```python
from build123d import *

# Parameters (mm, degrees)
EXTRUDE_1_DEPTH          = 99
CUT_EXTRUDE_1_DEPTH      = 102.247222184
CUT_EXTRUDE_1_DEPTH_BACK = 102.247222184
SKETCH_2_R               = 2
CUT_EXTRUDE_2_DEPTH      = 102.247222184
CUT_EXTRUDE_2_DEPTH_BACK = 102.247222184
SKETCH_3_R               = 2


with BuildPart() as part:
    # 草图1 → 凸台-拉伸1 (new, symmetric)
    with BuildSketch(Plane(origin=(0, 0, 0), x_dir=(1, 0, 0), z_dir=(0, 1, 0))):
        with BuildLine():
            Line((-11, -15), (11, -15))
            ThreePointArc((11, -15), (13.828427125, -13.828427125), (15, -11))
            Line((15, -11), (15, 11))
            ThreePointArc((15, 11), (13.828427125, 13.828427125), (11, 15))
            Line((11, 15), (-11, 15))
            ThreePointArc((-11, 15), (-13.828427125, 13.828427125), (-15, 11))
            Line((-15, 11), (-15, -11))
            ThreePointArc((-15, -11), (-13.828427125, -13.828427125), (-11, -15))
        make_face()
        with BuildLine():
            Line((-11, -13), (11, -13))
            ThreePointArc((11, -13), (12.414213562, -12.414213562), (13, -11))
            Line((13, -11), (13, 11))
            ThreePointArc((13, 11), (12.414213562, 12.414213562), (11, 13))
            Line((11, 13), (-11, 13))
            ThreePointArc((-11, 13), (-12.414213562, 12.414213562), (-13, 11))
            Line((-13, 11), (-13, -11))
            ThreePointArc((-13, -11), (-12.414213562, -12.414213562), (-11, -13))
        make_face(mode=Mode.SUBTRACT)
    extrude(amount=EXTRUDE_1_DEPTH, both=True)

    # 草图2 → 切除-拉伸1 (cut, two sides: drawn at the far end of the back side and taken through both)
    with BuildSketch(Plane(origin=(0, 0, 0), x_dir=(0, 0, -1), z_dir=(1, 0, 0)).offset(-CUT_EXTRUDE_1_DEPTH_BACK)):
        with Locations((8, 0)):
            Circle(SKETCH_2_R)
        with Locations((-8, 0)):
            Circle(SKETCH_2_R)
    extrude(amount=CUT_EXTRUDE_1_DEPTH + CUT_EXTRUDE_1_DEPTH_BACK, mode=Mode.SUBTRACT)

    # 草图3 → 切除-拉伸2 (cut, two sides: drawn at the far end of the back side and taken through both)
    with BuildSketch(Plane.XY.offset(-CUT_EXTRUDE_2_DEPTH_BACK)):
        with Locations((0, 84)):
            Circle(SKETCH_3_R)
        Circle(SKETCH_3_R)
        with Locations((0, -84)):
            Circle(SKETCH_3_R)
    extrude(amount=CUT_EXTRUDE_2_DEPTH + CUT_EXTRUDE_2_DEPTH_BACK, mode=Mode.SUBTRACT)


solid = part.part
```
Geometry: final body of the model. Coordinates: model frame, mm. A direction names the side the tool comes from. Round coordinates to 2 decimals unless told otherwise and drop trailing zeros. Order: outer loops, then holes, each group sorted by start corner. A loop starts at its lowest first (then second) coordinate and runs counter-clockwise, first axis right, second up. Notation, with made-up numbers: (68, 71.25) -> (113, 71.25) arc R25 cw to (113, 107.25) -> close; hole circle Ø11 at (83, 79). An arc over 180 degrees is marked (long way). Use CSV: the item, a comma, the result in double quotes. Start each with the question number.
1) Section A-A (x = 0). State how many separate pieces and enclosed holes the cut face has, and give its area (3 significant figures).
2) Material intervals for line 1 along Y through (x, z) = (0, 13.4); line 2 along Z through (x, y) = (-6, 35); line 3 along Y through (x, z) = (-14.4, -8), sorted ascending. Write a range as from..to.
3) Set-up query: faces 4 (the face through (-14, 0, -6)), 5 (the face through (-13, 1, 0)). Return all of +Z, -Z, +X, -X, +Y, -Y with unobstructed straight access to the full face (end or side cutting, diameter ignored); none if empty.
4) Section B-B (y = -5.5). Return the cut outline in (x, z).
5) Draft query along Y for faces 1 (the face through (-13.859, 1.386, 13.797)), 2 (the face through (-14, 99, 0)), 3 (the face through (-14, -1.2, 9.6)). Return one class per face: +Y half, -Y half, draft (parallel to the pull), parting line (faces both ways), or undercut.
6) Section C-C (z = -8). Return the cut outline in (x, y), and give its area (3 significant figures).
7) Section D-D (y = 84). Return the cut outline in (x, z), and give its area (3 significant figures).
Returned:
1,separate pieces,"8"
1,enclosed holes,"0"
1,area,"744 mm²"
2,line 1,"y = -99..-86, -82..-2, 2..82, 86..99"
2,line 2,"z = -15..-13, 13..15"
2,line 3,"y = -99..-2, 2..99"
3,face 4,"+X, -X"
3,face 5,"+Y, -Y"
4,outline,"(-15, -11) arc R4 ccw to (-11, -15) -> (11, -15) arc R4 ccw to (15, -11) -> (15, 11) arc R4 ccw to (11, 15) -> (-11, 15) arc R4 ccw to (-15, 11) -> close; hole (-13, -11) arc R2 ccw to (-11, -13) -> (11, -13) arc R2 ccw to (13, -11) -> (13, 11) arc R2 ccw to (11, 13) -> (-11, 13) arc R2 ccw to (-13, 11) -> close"
5,face 1,"draft"
5,face 2,"+Y half"
5,face 3,"undercut"
6,outline,"(-15, -99) -> (-13, -99) -> (-13, -2) -> (-15, -2) -> close; (-15, 2) -> (-13, 2) -> (-13, 99) -> (-15, 99) -> close; (13, -99) -> (15, -99) -> (15, -2) -> (13, -2) -> close; (13, 2) -> (15, 2) -> (15, 99) -> (13, 99) -> close"
6,area,"776 mm²"
7,outline,"(-15, -11) arc R4 ccw to (-11, -15) -> (-2, -15) -> (-2, -13) -> (-11, -13) arc R2 cw to (-13, -11) -> (-13, 11) arc R2 cw to (-11, 13) -> (-2, 13) -> (-2, 15) -> (-11, 15) arc R4 ccw to (-15, 11) -> close; (2, -15) -> (11, -15) arc R4 ccw to (15, -11) -> (15, 11) arc R4 ccw to (11, 15) -> (2, 15) -> (2, 13) -> (11, 13) arc R2 cw to (13, 11) -> (13, -11) arc R2 cw to (11, -13) -> (2, -13) -> close"
7,area,"198 mm²"
